Source: three-view drawing plus pictorial views. Frame: mm from the lowest corner of the part. A direction names the side the tool comes from. Round coordinates to 2 decimals unless told otherwise and drop trailing zeros. Order: outer loops, then holes, each group sorted by start corner. A loop starts at its lowest first (then second) coordinate and runs counter-clockwise, first axis right, second up. Notation, with made-up numbers: M 77,69.5 L 104,69.5 A31 ccw 104,108.5 Z; hole C -23,52 d11. An arc over 180 degrees is marked long. Return JSON: item names as keys, results as strings. Group by question number.
Q1. Ray query, probe 1 along X at (y, z) = (22.5, 76.2) (1 decimal); probe 2 along Y at (x, z) = (22, 81.5); probe 3 along Y at (x, z) = (18, 22). Return the intervals inside material, ascending.
Q2. Cut plane B-B on z = 67. Output: boundary loops of the cut face in (x, y).
Q3. Mould query, pull axis Y, two halves, no side actions, for the marked faces 4, 5 and 6. Classes: released by +Y, released by -Y, zero draft, split by the parting line, or undercut.
Q4. Contact query for flat-ended pins moving along their axis: pin 1 (11.5 mm diameter, centred on x = 11, z = 12.5, fed in from +Y); pin 2 (5.5 mm diameter, centred on x = 12.7, z = 31.75, fed in from -Y); pin 3 (10 mm diameter, centred on x = 3, z = 11, fed in from -Y); pin 4 (8 mm diameter, centred on x = 19, y = 5.5, fed in from +Z). Output: stop coordinate, or through.
Q5. Access query for the marked faces 1, 2 and 3. Directions: +Z, -Z, +X, -X, +Y, -Y. A direction counts if a zero-diameter tool reaches every point of the face in a straight line with its end or side. Return the directions, or none.
Q6. Cut plane A-A on x = 12.7. Count the separate pieces of the cut face and the enclosed holes in it, and give its area (3 significant figures).
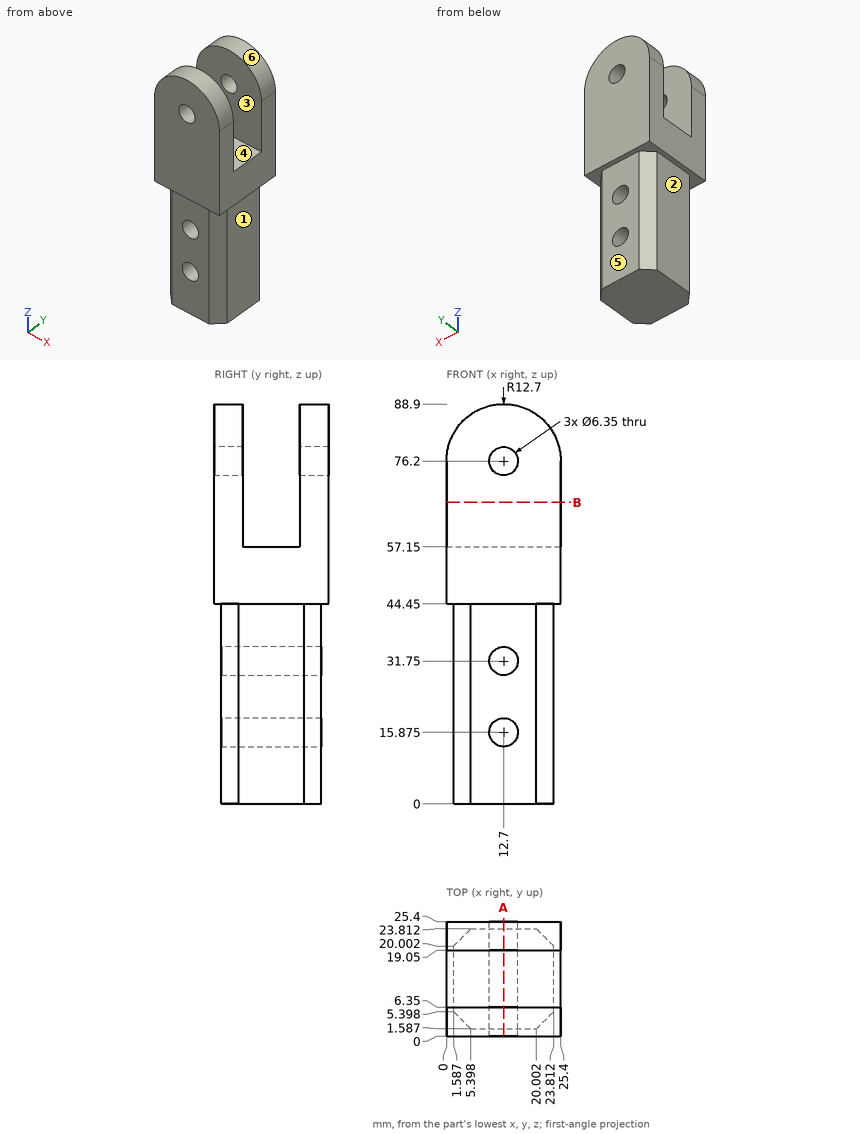
Result sheet:
{
 "1": {"probe 1": "x = 0 to 9.5, 15.9 to 25.4", "probe 2": "y = 0 to 6.35, 19.05 to 25.4", "probe 3": "y = 1.59 to 23.81"},
 "2": {"outline": "M 0,0 L 25.4,0 L 25.4,6.35 L 0,6.35 Z; M 0,19.05 L 25.4,19.05 L 25.4,25.4 L 0,25.4 Z"},
 "3": {"face 4": "undercut", "face 5": "released by +Y", "face 6": "zero draft"},
 "4": {"pin 1": "stops at y = 23.81", "pin 2": "passes through", "pin 3": "stops at y = 1.59", "pin 4": "stops at z = 88.69"},
 "5": {"face 1": "-Z, +X, +Y, -Y", "face 2": "-Z, -X, +Y, -Y", "face 3": "+Z, +X, -X"},
 "6": {"separate pieces": "5", "enclosed holes": "0", "area": "1,350 mm²"}
}
